from build123d import *

# Parameters (mm, degrees)
SKETCH2_W                = 20
SKETCH2_H                = 10
BOSS_EXTRUDE1_DEPTH      = 11
SKETCH3_W                = 20
SKETCH3_H                = 2
BOSS_EXTRUDE2_DEPTH      = 3
BOSS_EXTRUDE2_DEPTH_BACK = 13
SKETCH4_W                = 12
SKETCH4_H                = 40
BOSS_EXTRUDE3_DEPTH      = 1
SKETCH5_W                = 2
SKETCH5_H                = 60
BOSS_EXTRUDE4_DEPTH      = 45
F_4_0MM_DOWEL_SLOT1_D    = 4
F_8_0MM_DOWEL_SLOT4_D    = 8
SKETCH22_W               = 9.202465877
SKETCH22_H               = 9.167340884
BOSS_EXTRUDE5_DEPTH      = 0.001
BOSS_EXTRUDE5_DEPTH_BACK = 30
CUT_EXTRUDE1_DEPTH       = 31
F_2_5MM_DOWEL_SLOT1_D    = 2.5
CUT_EXTRUDE2_DEPTH       = 10
CUT_EXTRUDE3_DEPTH       = 10
FILLET1_R                = 10


with BuildPart() as part:
    # Sketch2 → Boss-Extrude1 (new body)
    with BuildSketch(Plane.XY):
        Rectangle(SKETCH2_W, SKETCH2_H)
    extrude(amount=BOSS_EXTRUDE1_DEPTH)

    # Sketch3 → Boss-Extrude2 (add, two sides)
    with BuildSketch(Plane(origin=(0, 5, 0), x_dir=(1, 0, 0), z_dir=(0, 1, 0))) as boss_extrude2_sk:
        with Locations((0, -2.5)):
            Rectangle(SKETCH3_W, SKETCH3_H)
    extrude(amount=BOSS_EXTRUDE2_DEPTH)
    extrude(boss_extrude2_sk.sketch, amount=-BOSS_EXTRUDE2_DEPTH_BACK)

    # Sketch4 → Boss-Extrude3 (add)
    with BuildSketch(Plane(origin=(10, 0, 0), x_dir=(0, 0, -1), z_dir=(1, 0, 0))):
        with Locations((-5, 0)):
            Rectangle(SKETCH4_W, SKETCH4_H)
    extrude(amount=BOSS_EXTRUDE3_DEPTH)

    # Sketch5 → Boss-Extrude4 (add)
    with BuildSketch(Plane(origin=(11, 0, 0), x_dir=(0, 0, -1), z_dir=(1, 0, 0))):
        with Locations((0, 10)):
            Rectangle(SKETCH5_W, SKETCH5_H)
    extrude(amount=BOSS_EXTRUDE4_DEPTH)

    # Ø4.0mm Dowel Slot1 (through all)
    with Locations(Plane.XY.offset(1)):
        with Locations((16, 18), (51, 18)):
            Hole(F_4_0MM_DOWEL_SLOT1_D / 2)

    # Ø8.0mm Dowel Slot4 (through all)
    with Locations(Plane.XY.offset(1)):
        with Locations((33.5, 26)):
            Hole(F_8_0MM_DOWEL_SLOT4_D / 2)

    # Sketch22 → Boss-Extrude5 (add, two sides)
    with BuildSketch(Plane(origin=(11, -20, 1), x_dir=(-1, 0, 0), z_dir=(0, -1, 0))) as boss_extrude5_sk:
        with Locations((-4.601232938, -4.583670442)):
            Rectangle(SKETCH22_W, SKETCH22_H)
    extrude(amount=BOSS_EXTRUDE5_DEPTH)
    extrude(boss_extrude5_sk.sketch, amount=-BOSS_EXTRUDE5_DEPTH_BACK)

    # Sketch23 → Cut-Extrude1 (cut)
    with BuildSketch(Plane(origin=(0, 10, 0), x_dir=(1, 0, 0), z_dir=(0, 1, 0))):
        Polygon((20.202465877, -1), (11, -10.167340884), (20.202465877, -10.167340884), align=None)
    extrude(amount=-CUT_EXTRUDE1_DEPTH, mode=Mode.SUBTRACT)

    # Ø2.5mm Dowel Slot1 (through all)
    with Locations(Plane.XY.offset(11)):
        with Locations((-5.633536512, 0), (5.798014949, 0)):
            Hole(F_2_5MM_DOWEL_SLOT1_D / 2)

    # Sketch26 → Cut-Extrude2 (cut)
    with BuildSketch(Plane.XY.offset(1)):
        Polygon((29.003862236, 40), (11, 25.763222488), (11, 40), align=None)
        Polygon((56, 40), (39.686791896, 40), (56, 23.686791896), align=None)
    extrude(amount=-CUT_EXTRUDE2_DEPTH, mode=Mode.SUBTRACT)

    # Sketch27 → Cut-Extrude3 (cut)
    with BuildSketch(Plane.XY.offset(1)):
        Polygon((32.71386297, -20), (56, -1.611523644), (56, -20), align=None)
    extrude(amount=-CUT_EXTRUDE3_DEPTH, mode=Mode.SUBTRACT)

    # Fillet1
    fillet1_edges = [part.edges().sort_by_distance(p)[0] for p in [
        (29.003862236, 40, 0),
        (11, 25.763222488, 0),
        (56, 23.686791896, 0),
        (39.686791896, 40, 0),
        (56, -1.611523644, 0),
    ]]
    fillet(fillet1_edges, radius=FILLET1_R)


solid = part.part
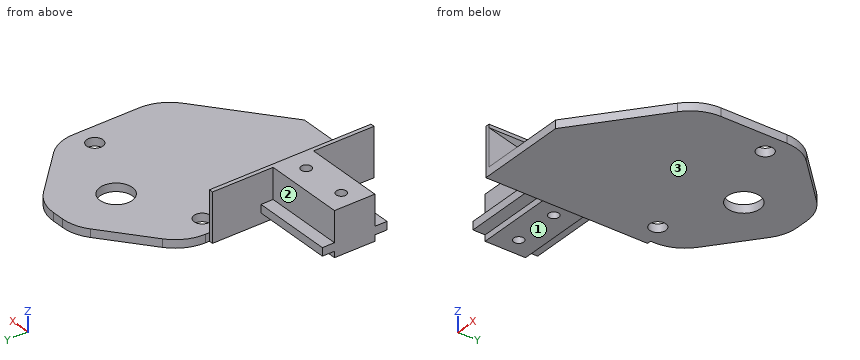
Geometry: final body of the model. Coordinates: model frame, mm. Face numbers are marked on the shaded views. A direction names the side the tool comes from. Coordinates: 2 decimals unless noted, no trailing zeros. Write each loop counter-clockwise with the first axis right and the second up, starting at its lowest first coordinate (ties: lowest second). Pieces come first, ordered by that corner, then holes. Notation, with made-up numbers: (44.25, 8.5) - (97.25, 8.5) arc R15 ccw to (97.25, 12.5) - close; hole circle Ø1 at (84.5, 89.5). An arc over 180 degrees is marked (long way). Return JSON: item names as keys, results as strings.
Item 1: Pin query (flat end, axial travel): pin 1 Ø1.5 at (y, z) = (13.5, 8) entering from -X; pin 2 Ø8 at (x, y) = (2, 0.5) entering from -Z; pin 3 Ø2 at (y, z) = (-4.5, 7.5) entering from +X. Return the tip coordinate at first contact, or that it passes through.
Completed:
{"pin 1": "stops at x = 10", "pin 2": "stops at z = 0", "pin 3": "stops at x = 14.68"}
Item 2: Section query B-B (z = 6.25). Count the separate pieces of the cut face and the enclosed holes in it, and give its area (3 significant figures).
Completed:
{"separate pieces": "1", "enclosed holes": "2", "area": "348 mm2"}
Item 3: Line query: L1, parallel to X at y = -1, z = 6.25; L2, parallel to X at y = 17, z = 2.5; L3, parallel to Z at x = 34, y = -1.5. Output: solid intervals per line, ascending.
Completed:
{"L1": "x = -10 to -6.38, -4.88 to 5.05, 6.55 to 14.93", "L2": "x = 10 to 11", "L3": "z = -1 to 1"}
Item 4: Section query A-A (y = 18). Output: boundary loops of the cut face in (x, z).
Completed:
{"outline": "(10, -1) - (14, -1) - (14, 1) - (11, 1) - (11, 11) - (10, 11) - close; (18, -1) - (49, -1) - (49, 1) - (18, 1) - close; (53, -1) - (56, -1) - (56, 1) - (53, 1) - close"}
Item 5: Section query C-C (x = 33.5). Output: boundary loops of the cut face in (y, z), and give its area (3 significant figures).
Completed:
{"outline": "(-19.38, -1) - (22, -1) - (22, 1) - (-19.38, 1) - close; (30, -1) - (40, -1) - (40, 1) - (30, 1) - close", "area": "103 mm2"}
Item 6: Section query D-D (y = -9.5). Output: boundary loops of the cut face in (x, z), and give its area (3 significant figures).
Completed:
{"outline": "(10, -1) - (46.01, -1) - (46.01, 1) - (20.2, 1) - (11, 10.17) - (11, 11) - (10, 11) - close", "area": "124 mm2"}
Item 7: Reachability of the marked faces 1, 2 and 3 from +Z, -Z, +X, -X, +Y, -Y: full face, straight path, thin tool, end or side. Return the list, or none.
Completed:
{"face 1": "-Z, -X, +Y, -Y", "face 2": "+Z, -X, +Y", "face 3": "-Z, +X, -X, +Y, -Y"}
